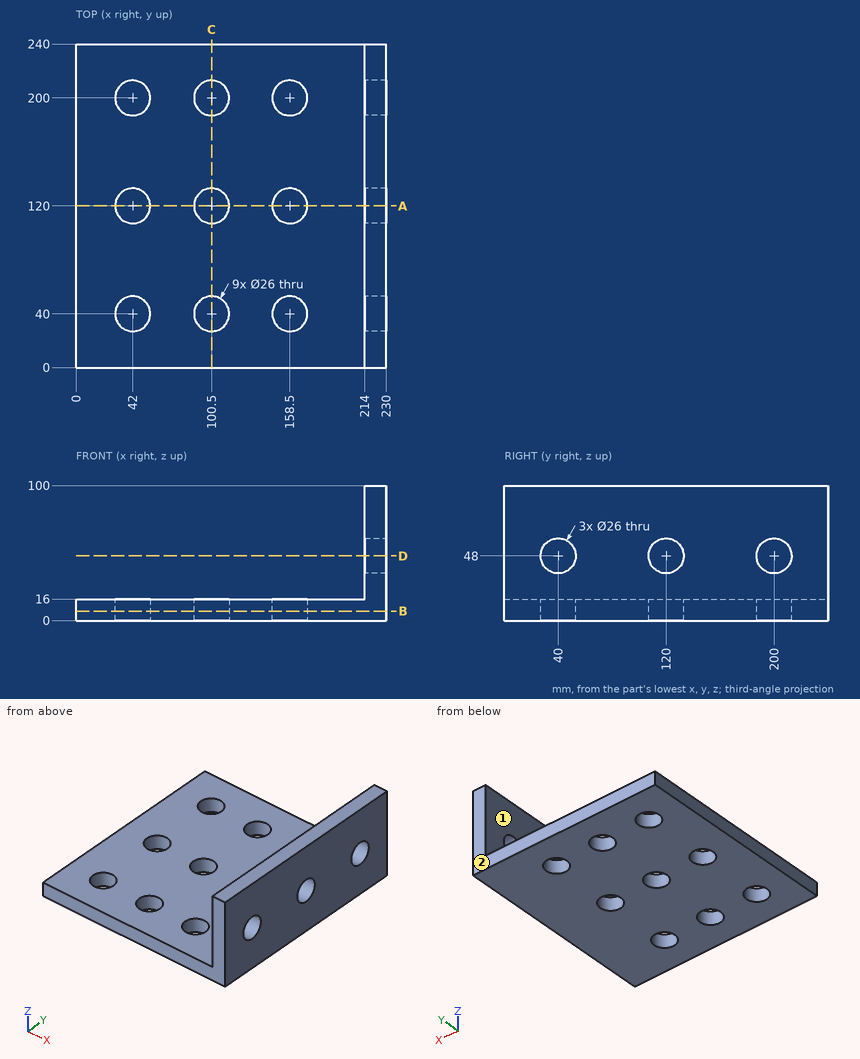
Study the drawing (mm; zero at the part's minimum x, y, z) and answer. A direction names the side the tool comes from. Coordinates: 2 decimals unless noted, no trailing zeros. Loops run counter-clockwise (first coordinate to the right, second up) from the corner with the lowest first, then second, coordinate; pieces in that order, holes last. Notation, with made-up numbers: M 30,62.5 L 49,62.5 A18 cw 49,73.5 Z; hole C -24.5,10 d2. An arc over 180 degrees is marked long. Answer in a Markdown table with one row per item. Add a question column.
1. Find section B-B, the plane z = 7. State how many separate pieces and enclosed holes the cut face has, then the cut area to 3 significant figures.
2. Find section A-A, the plane y = 120. Write down the section's boundary in (x, z), then the cut area to 3 significant figures.
3. Find section C-C, the plane x = 100.5. Write down the section's boundary in (y, z), then the cut area to 3 significant figures.
4. A flat-ended cylindrical pin translates along its axis: P1, Ø3, axis at y = 32, z = 66, coming from the -X side. Find the tip coordinate at first contact, or state that the pin passes through.
5. Consider L1, parallel to Y at x = 100.5, z = 5.25; L2, parallel to Z at x = 53, y = 207; L3, parallel to X at y = 73.5, z = 21. Determine where each line is inside the solid, lowest interval first.
6. A tool of negligible diameter and unlimited length cuts with its end or side. For the marked faces 1 and 2, from which of +Z, -Z, +X, -X, +Y, -Y can it reach the whole face along a straight path? Write none if from no direction.
7. Find section D-D, the plane z = 48. Write down the section's boundary in (x, y).
Reported:
| question | item | result |
|---|---|---|
| 1 | separate pieces | 1 |
| 1 | enclosed holes | 9 |
| 1 | area | 50,400 mm^2 |
| 2 | outline | M 0,0 L 29,0 L 29,16 L 0,16 Z; M 55,0 L 87.5,0 L 87.5,16 L 55,16 Z; M 113.5,0 L 145.5,0 L 145.5,16 L 113.5,16 Z; M 171.5,0 L 230,0 L 230,35 L 214,35 L 214,16 L 171.5,16 Z; M 214,61 L 230,61 L 230,100 L 214,100 Z |
| 2 | area | 3,360 mm^2 |
| 3 | outline | M 0,0 L 27,0 L 27,16 L 0,16 Z; M 53,0 L 107,0 L 107,16 L 53,16 Z; M 133,0 L 187,0 L 187,16 L 133,16 Z; M 213,0 L 240,0 L 240,16 L 213,16 Z |
| 3 | area | 2,590 mm^2 |
| 4 | P1 | stops at x = 214 |
| 5 | L1 | y = 0 to 27, 53 to 107, 133 to 187, 213 to 240 |
| 5 | L2 | z = 0 to 16 |
| 5 | L3 | x = 214 to 230 |
| 6 | face 1 | +Z, -X, +Y, -Y |
| 6 | face 2 | +Z, -Z, +X, -X, +Y |
| 7 | outline | M 214,0 L 230,0 L 230,27 L 214,27 Z; M 214,53 L 230,53 L 230,107 L 214,107 Z; M 214,133 L 230,133 L 230,187 L 214,187 Z; M 214,213 L 230,213 L 230,240 L 214,240 Z |
